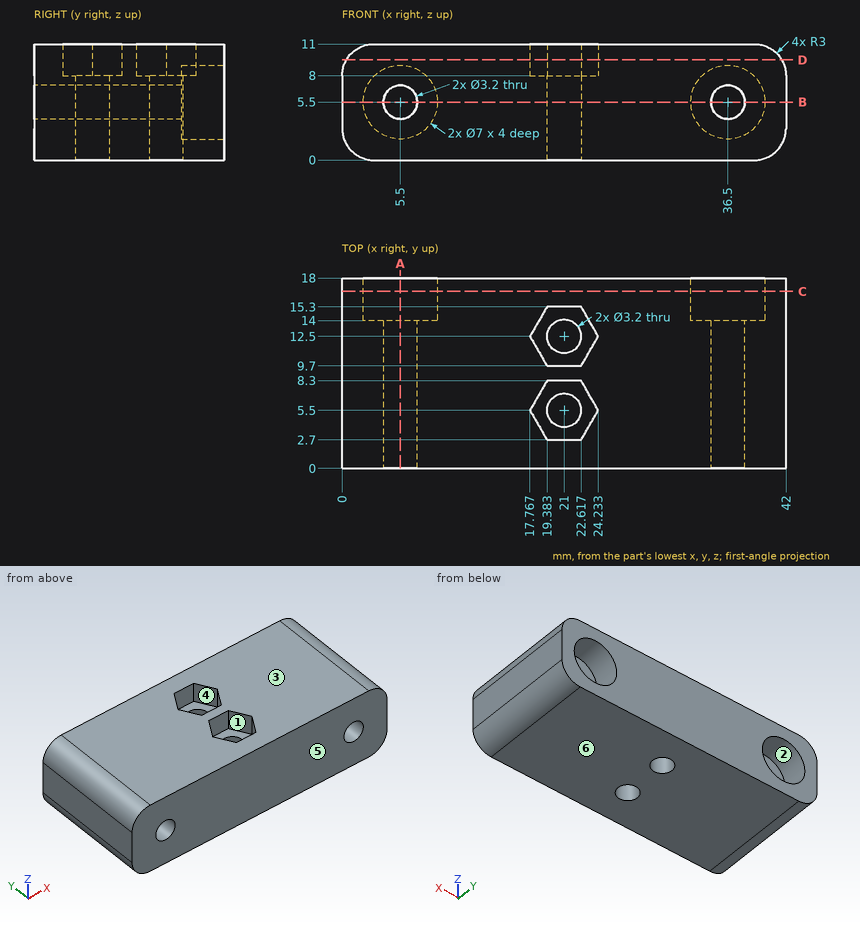
Can you work these out from the drawing? Everything is in mm from the part's minimum corner. A direction names the side the tool comes from. Give positions to 0.01 mm unless a question says otherwise; leave off trailing zeros. Loops run counter-clockwise (first coordinate to the right, second up) from the corner with the lowest first, then second, coordinate; pieces in that order, holes last. Notation, with made-up numbers: (-29, -29) -> (-2, -29) arc R13 cw to (-2, -22) -> close; hole circle Ø2 at (-12.75, 26.25). An arc over 180 degrees is marked (long way). Return JSON: item names as keys, results as strings.
Q1. I want a section at C-C, the plane y = 16.75. List the corners of the cut face in (x, z) for me, then the cut area to 3 significant figures.
Checks:
{"outline": "(0, 3) arc R3 ccw to (3, 0) -> (39, 0) arc R3 ccw to (42, 3) -> (42, 8) arc R3 ccw to (39, 11) -> (3, 11) arc R3 ccw to (0, 8) -> close; hole circle Ø7 at (5.5, 5.5); hole circle Ø7 at (36.5, 5.5)", "area": "377 mm2"}
Q2. I want a section at B-B, the plane z = 5.5. List the corners of the cut face in (x, y) for me.
Checks:
{"outline": "(0, 0) -> (3.9, 0) -> (3.9, 14) -> (2, 14) -> (2, 18) -> (0, 18) -> close; (7.1, 0) -> (34.9, 0) -> (34.9, 14) -> (33, 14) -> (33, 18) -> (9, 18) -> (9, 14) -> (7.1, 14) -> close; (38.1, 0) -> (42, 0) -> (42, 18) -> (40, 18) -> (40, 14) -> (38.1, 14) -> close; hole circle Ø3.2 at (21, 5.5); hole circle Ø3.2 at (21, 12.5)"}
Q3. We'd pull the mould along Y, two halves only. Please class the marked faces 4, 5 and 6: released by +Y, released by -Y, zero draft, split by the parting line, or undercut.
Checks:
{"face 4": "undercut", "face 5": "released by -Y", "face 6": "zero draft"}
Q4. On a 3-axis mill with a long thin cutter (end or side, diameter ignored), from which of +Z, -Z, +X, -X, +Y, -Y can I reach the whole of each face in a straight line? I mean the marked faces 1, 2 and 3. Say none if no direction works.
Checks:
{"face 1": "+Z", "face 2": "+Y", "face 3": "+Z, +X, -X, +Y, -Y"}
Q5. I want a section at A-A, the plane x = 5.5. List the corners of the cut face in (y, z) for me, then the cut area to 3 significant figures.
Checks:
{"outline": "(0, 0) -> (18, 0) -> (18, 2) -> (14, 2) -> (14, 3.9) -> (0, 3.9) -> close; (0, 7.1) -> (14, 7.1) -> (14, 9) -> (18, 9) -> (18, 11) -> (0, 11) -> close", "area": "125 mm2"}
Q6. I want a section at D-D, the plane z = 9.5. List the corners of the cut face in (x, y) for me.
Checks:
{"outline": "(0.4, 0) -> (41.6, 0) -> (41.6, 18) -> (0.4, 18) -> close; hole (17.77, 5.5) -> (19.38, 2.7) -> (22.62, 2.7) -> (24.23, 5.5) -> (22.62, 8.3) -> (19.38, 8.3) -> close; hole (17.77, 12.5) -> (19.38, 9.7) -> (22.62, 9.7) -> (24.23, 12.5) -> (22.62, 15.3) -> (19.38, 15.3) -> close"}
Q7. For pin 1 Ø2 at (x, z) = (37.5, 4) entering from +Y; pin 2 Ø3.5 at (x, y) = (21, 12.5) entering from +Z, each with a flat end and sliding along its axis, tell me the tip position at first contact or that it passes through.
Checks:
{"pin 1": "stops at y = 14", "pin 2": "stops at z = 8"}
Q8. I need wall thicknesses on probe 1 along X at (y, z) = (7.5, 5.5); probe 2 along X at (y, z) = (15.45, 5.5); probe 3 along X at (y, z) = (11.75, 5) (1 decimal). Which ranges of each line are inside material? Lowest first, please.
Checks:
{"probe 1": "x = 0 to 3.9, 7.1 to 34.9, 38.1 to 42", "probe 2": "x = 0 to 2, 9 to 33, 40 to 42", "probe 3": "x = 0 to 4, 7 to 19.6, 22.4 to 35, 38 to 42"}
